Read the model definition and answer for the solid it produces. Units are mm, in the model's axes. Face numbers are marked on the shaded views. A direction names the side the tool comes from. Give positions to 0.01 mm unless a question says otherwise; leave off trailing zeros. Loops run counter-clockwise (first coordinate to the right, second up) from the corner with the lowest first, then second, coordinate; pieces in that order, holes last.
(1) Find section A-A, the plane x = 173. Write down the section's boundary in (y, z).
(2) Straight lines are drawn through the part: probe 1 along Y at (x, z) = (144.5, 27); probe 2 along X at (y, z) = (86, -16.5); probe 3 along X at (y, z) = (164, -5.5). For each, find the intervals that lie inside material, in ascending order.
(3) Find section B-B, the plane z = 29. Write down the section's boundary in (x, y).
(4) Each of these flat-tipped pins is pushed along its axis until it touches: P1, Ø1.8, axis at x = 219.5, z = 6.5, coming from the -Y side; P2, Ø5, axis at x = 220.5, z = 18, coming from the +Y side. Where does it stop, or does it pass through?
(5) Find section C-C, the plane y = 98.5. Write down the section's boundary in (x, z), then the cut area to 3 significant figures.
(6) Which of the six approach directions +Z, -Z, +X, -X, +Y, -Y give full straight-line access (tool end or side, diameter ignored) to the marked faces 1 and 2?
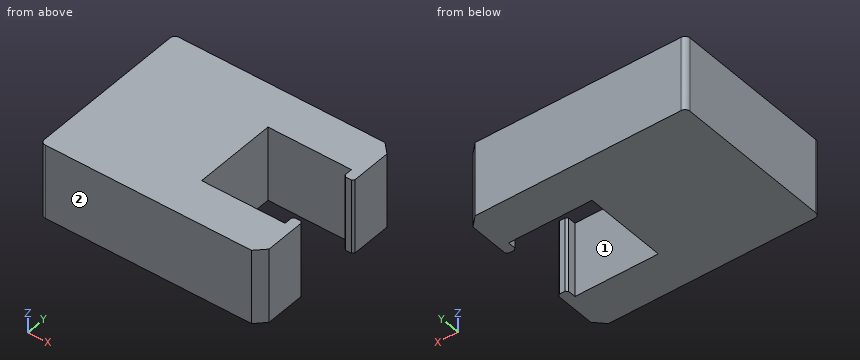
```python
from build123d import *

# Parameters (mm, degrees)
BOSS_EXTRUDE1_DEPTH = 38.1
CHAMFER1_SIZE       = 10
CHAMFER2_SIZE       = 2
FILLET1_R           = 5


with BuildPart() as part:
    # Sketch1 → Boss-Extrude1 (new, symmetric)
    with BuildSketch(Plane.XY):
        Polygon((0, 0), (225, 0), (225, 53), (215, 53), (215, 43), (130, 43), (130, 128), (215, 128), (215, 118), (225, 118), (225, 171), (0, 171), align=None)
    extrude(amount=BOSS_EXTRUDE1_DEPTH, both=True)

    # Chamfer1
    chamfer1_edges = [part.edges().sort_by_distance(p)[0] for p in [
        (225, 171, 0),
        (225, 0, 0),
    ]]
    chamfer(chamfer1_edges, length=CHAMFER1_SIZE)

    # Chamfer2
    chamfer2_edges = [part.edges().sort_by_distance(p)[0] for p in [
        (225, 118, 0),
        (215, 118, 0),
        (215, 53, 0),
        (225, 53, 0),
    ]]
    chamfer(chamfer2_edges, length=CHAMFER2_SIZE)

    # Fillet1
    fillet1_edges = [part.edges().sort_by_distance(p)[0] for p in [
        (0, 171, 0),
        (0, 0, 0),
    ]]
    fillet(fillet1_edges, radius=FILLET1_R)


solid = part.part
```
Entries:
1. outline: (0, -38.1) - (43, -38.1) - (43, 38.1) - (0, 38.1) - close; (128, -38.1) - (171, -38.1) - (171, 38.1) - (128, 38.1) - close
2. probe 1: y = 0 to 43, 128 to 171
2. probe 2: x = 0 to 130
2. probe 3: x = 0 to 222
3. outline: (0, 5) arc R5 ccw to (5, 0) - (215, 0) - (225, 10) - (225, 51) - (223, 53) - (217, 53) - (215, 51) - (215, 43) - (130, 43) - (130, 128) - (215, 128) - (215, 120) - (217, 118) - (223, 118) - (225, 120) - (225, 161) - (215, 171) - (5, 171) arc R5 ccw to (0, 166) - close
4. P1: stops at y = 3.6
4. P2: stops at y = 168
5. outline: (0, -38.1) - (130, -38.1) - (130, 38.1) - (0, 38.1) - close
5. area: 9,910 mm2
6. face 1: +Z, -Z
6. face 2: +Z, -Z, +X, -X, -Y
